Geometry: final body of the model. Coordinates: model frame, mm. Face numbers are marked on the shaded views. A direction names the side the tool comes from. Give positions to 0.01 mm unless a question says otherwise; leave off trailing zeros. Write each loop counter-clockwise with the first axis right and the second up, starting at its lowest first coordinate (ties: lowest second). Pieces come first, ordered by that corner, then holes. Notation, with made-up numbers: M 85,43 L 93,43 A25 ccw 93,67 Z; hole C 34,-2 d8. An arc over 180 degrees is marked long. Answer as a JSON object with one key per item and string values.
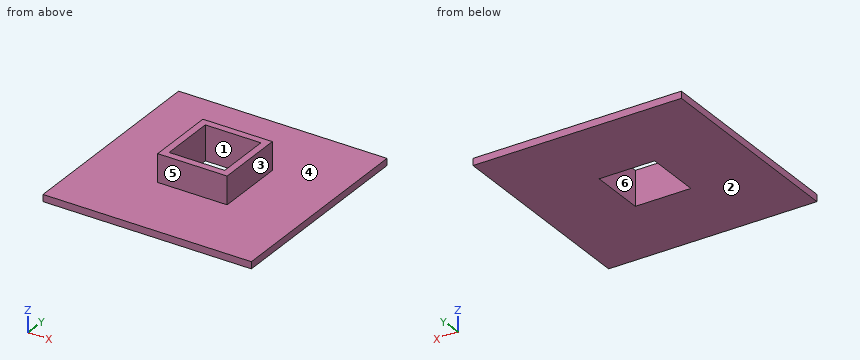
from build123d import *

# Parameters (mm, degrees)
BOX002_W     = 16
BOX002_H     = 16
BOX002_DEPTH = 10
BOX003_W     = 20
BOX003_H     = 20
BOX003_DEPTH = 10
BOX001_W     = 16
BOX001_H     = 16
BOX001_DEPTH = 3
BOX_W        = 60
BOX_H        = 60
BOX_DEPTH    = 2


with BuildPart() as cube002:
    # Box002 → Box002 (new body)
    with BuildSketch(Plane(origin=(-8, -8, 0), x_dir=(1, 0, 0), z_dir=(0, 0, 1))):
        with Locations((8, 8)):
            Rectangle(BOX002_W, BOX002_H)
    extrude(amount=BOX002_DEPTH)


with BuildPart() as cut001:
    # Box003 → Box003 (new body)
    with BuildSketch(Plane(origin=(-10, -10, 0), x_dir=(1, 0, 0), z_dir=(0, 0, 1))):
        with Locations((10, 10)):
            Rectangle(BOX003_W, BOX003_H)
    extrude(amount=BOX003_DEPTH)

    # Cut001: cut Cube002
    add(cube002.part, mode=Mode.SUBTRACT)


with BuildPart() as cube001:
    # Box001 → Box001 (new body)
    with BuildSketch(Plane(origin=(-8, -8, 0), x_dir=(1, 0, 0), z_dir=(0, 0, 1))):
        with Locations((8, 8)):
            Rectangle(BOX001_W, BOX001_H)
    extrude(amount=BOX001_DEPTH)


with BuildPart() as fusion:
    # Box → Box (new body)
    with BuildSketch(Plane(origin=(-30, -30, 0), x_dir=(1, 0, 0), z_dir=(0, 0, 1))):
        with Locations((30, 30)):
            Rectangle(BOX_W, BOX_H)
    extrude(amount=BOX_DEPTH)

    # Cut: cut Cube001
    add(cube001.part, mode=Mode.SUBTRACT)

    # Fusion: union Cut001
    add(cut001.part)


solid = fusion.part
1) Pull-direction query (Y, two-part tool) for the marked faces 4, 5 and 6; classes: pulls with the +Y half, pulls with the -Y half, needs draft (parallel to the pull), parting line crosses it, or undercut.
Geometry check:
{"face 4": "needs draft", "face 5": "pulls with the -Y half", "face 6": "undercut"}
2) Contact query for flat-ended pins moving along their axis: P1, Ø1, axis at x = 19.5, y = -3, coming from the +Z side; P2, Ø1.5, axis at x = -12.5, z = 6.5, coming from the +Y side (3 decimals); P3, Ø2.5, axis at x = -4.5, z = 4.5, coming from the +Y side; P4, Ø2.5, axis at x = 0.5, z = 5.5, coming from the -Y side. Output: stop coordinate, or through.
Geometry check:
{"P1": "stops at z = 2", "P2": "passes through", "P3": "stops at y = 10", "P4": "stops at y = -10"}
3) Line query: line 1 (Y direction, x = -1, z = 7.5); line 2 (Z direction, x = -25.5, y = 14). Output: solid intervals per line, ascending. Write a range as from..to.
Geometry check:
{"line 1": "y = -10..-8, 8..10", "line 2": "z = 0..2"}
4) Cut plane A-A on x = 6.5. Return loops of the section in (y, z), and give its area (3 significant figures).
Geometry check:
{"outline": "M -30,0 L -8,0 L -8,10 L -10,10 L -10,2 L -30,2 Z; M 8,0 L 30,0 L 30,2 L 10,2 L 10,10 L 8,10 Z", "area": "120 mm2"}
5) Cut plane D-D on z = 8.75. Return loops of the section in (x, y).
Geometry check:
{"outline": "M -10,-10 L 10,-10 L 10,10 L -10,10 Z; hole M -8,-8 L 8,-8 L 8,8 L -8,8 Z"}
6) Cut plane B-B on z = 1. Return loops of the section in (x, y).
Geometry check:
{"outline": "M -30,-30 L 30,-30 L 30,30 L -30,30 Z; hole M -8,-8 L 8,-8 L 8,8 L -8,8 Z"}
7) Set-up query: the marked faces 1, 2 and 3. Return all of +Z, -Z, +X, -X, +Y, -Y with unobstructed straight access to the full face (end or side cutting, diameter ignored); none if empty.
Geometry check:
{"face 1": "+Z, -Z", "face 2": "-Z, +X, -X, +Y, -Y", "face 3": "+Z, +X, +Y, -Y"}
